Could you check a few things on this model? Use its own coordinates, in mm. A direction names the side the tool comes from. Round coordinates to 2 decimals unless told otherwise and drop trailing zeros. Write each loop counter-clockwise with the first axis right and the second up, starting at its lowest first coordinate (ties: lowest second). Pieces come first, ordered by that corner, then holes. Notation, with made-up numbers: (35.5, 7) -> (51.5, 7) arc R22 cw to (51.5, 46) -> close; hole circle Ø10 at (33.5, 69.5). An arc over 180 degrees is marked (long way). Answer in a Markdown table with one row per item. Add a question column.
```python
from build123d import *

# Parameters (mm, degrees)
F0_R     = 2
F1_DEPTH = 40
F3_DEPTH = 5
F5_DEPTH = 10
F6_W     = 0.9371294279
F6_H     = 2
F6_W_2   = 0.6703293088
F6_W_3   = 1
F7_DEPTH = 25


with BuildPart() as f1:
    # F0 (on Top) → F1 (new body)
    with BuildSketch(Plane.XY):
        Circle(F0_R)
    extrude(amount=F1_DEPTH)

    # F2 (on face) → F3 (join)
    with BuildSketch(Plane.XY.offset(40)):
        with BuildLine():
            Line((0, 2), (-1.1547005384, 2))
            Line((-1.1547005384, 2), (-1.7320507826, 1.0000000433))
            ThreePointArc((-1.7320507826, 1.0000000433), (-0.9999999783, 1.7320508201), (0, 2))
        make_face()
        with BuildLine():
            ThreePointArc((-1.7320507826, -1.0000000433), (-2, 0), (-1.7320507826, 1.0000000433))
            Line((-1.7320507826, 1.0000000433), (-2.3094010768, 0))
            Line((-2.3094010768, 0), (-1.7320507826, -1.0000000433))
        make_face()
        with BuildLine():
            ThreePointArc((0, -2), (-0.9999999783, -1.7320508201), (-1.7320507826, -1.0000000433))
            Line((-1.7320507826, -1.0000000433), (-1.1547005384, -2))
            Line((-1.1547005384, -2), (0, -2))
        make_face()
        with BuildLine():
            ThreePointArc((1.7320507983, -1.0000000161), (0.999999992, -1.7320508122), (0, -2))
            Line((0, -2), (1.1547005384, -2))
            Line((1.1547005384, -2), (1.7320507983, -1.0000000161))
        make_face()
        with BuildLine():
            Line((2.3094010768, 0), (1.7320507826, 1.0000000433))
            ThreePointArc((1.7320507826, 1.0000000433), (1.9318516461, 0.5176381144), (2, 0))
            ThreePointArc((2, 0), (1.9318516502, -0.5176380992), (1.7320507983, -1.0000000161))
            Line((1.7320507983, -1.0000000161), (2.3094010768, 0))
        make_face()
        with BuildLine():
            Line((1.1547005384, 2), (0, 2))
            ThreePointArc((0, 2), (0.9999999783, 1.7320508201), (1.7320507826, 1.0000000433))
            Line((1.7320507826, 1.0000000433), (1.1547005384, 2))
        make_face()
        with BuildLine():
            ThreePointArc((1.7320507826, 1.0000000433), (0.9999999783, 1.7320508201), (0, 2))
            ThreePointArc((0, 2), (-0.9999999783, 1.7320508201), (-1.7320507826, 1.0000000433))
            ThreePointArc((-1.7320507826, 1.0000000433), (-2, 0), (-1.7320507826, -1.0000000433))
            ThreePointArc((-1.7320507826, -1.0000000433), (-0.9999999783, -1.7320508201), (0, -2))
            ThreePointArc((0, -2), (0.999999992, -1.7320508122), (1.7320507983, -1.0000000161))
            ThreePointArc((1.7320507983, -1.0000000161), (1.9318516502, -0.5176380992), (2, 0))
            ThreePointArc((2, 0), (1.9318516461, 0.5176381144), (1.7320507826, 1.0000000433))
        make_face()
    extrude(amount=F3_DEPTH)

    # F4 (on face) → F5 (join)
    with BuildSketch(Plane(origin=(0, 0, 0), x_dir=(1, 0, 0), z_dir=(0, 0, -1))):
        with BuildLine():
            ThreePointArc((1.1, 1.6703293088), (0.5741695665, 1.915810353), (0, 2))
            ThreePointArc((0, 2), (-0.5741695665, 1.915810353), (-1.1, 1.6703293088))
            Line((-1.1, 1.6703293088), (-1.1, -1.6703293088))
            ThreePointArc((-1.1, -1.6703293088), (-0.5741695665, -1.915810353), (0, -2))
            ThreePointArc((0, -2), (0.5741695665, -1.915810353), (1.1, -1.6703293088))
            Line((1.1, -1.6703293088), (1.1, 1.6703293088))
        make_face()
    extrude(amount=F5_DEPTH)

    # F6 (on face) → F7 (cut)
    with BuildSketch(Plane.YZ.offset(1.1)):
        with Locations((-2.1388940228, -4.197623184)):
            Rectangle(F6_W, F6_H)
        with Locations((-1.3351646544, -4.197623184)):
            Rectangle(F6_W_2, F6_H)
        with Locations((-0.5, -4.197623184)):
            Rectangle(F6_W_3, F6_H)
        with BuildLine():
            Line((1, -3.197623184), (0, -3.197623184))
            Line((0, -3.197623184), (0, -5.197623184))
            Line((0, -5.197623184), (-1, -5.197623184))
            Line((-1, -5.197623184), (-1, -6.7451779507))
            ThreePointArc((-1, -6.7451779507), (-0.7071067812, -7.4522847319), (0, -7.7451779507))
            ThreePointArc((0, -7.7451779507), (0.7071067812, -7.4522847319), (1, -6.7451779507))
            Line((1, -6.7451779507), (1, -3.197623184))
        make_face()
    extrude(amount=-F7_DEPTH, mode=Mode.SUBTRACT)


solid = f1.part
```
(1) On a 3-axis mill with a long thin cutter (end or side, diameter ignored), from which of +Z, -Z, +X, -X, +Y, -Y can I reach the whole of each face in a straight line? I mean faces 1 (the face through (-1.1, 1.5, -4.9)), 2 (the face through (0, 0, -3.198)), 3 (the face through (1.4, 0, 0)), 4 (the face through (0, -1, -6)). Say none if no direction works.
(2) Suppose I cut it at A-A, the plane z = 10. Please give me the cut outline in (x, y).
(3) If we mould it in two halves opening along Y, with no side actions, what happens to faces 5 (the face through (0, 1, -5)), 6 (the face through (-1.5, 0, 0)), 7 (the face through (0, 2, 42)), 8 (the face through (0, -2, 42))? For each: pulls with the +Y half, pulls with the -Y half, needs draft (parallel to the pull), parting line crosses it, or undercut.
(4) For P1, Ø1.2, axis at x = 0.5, z = -6, coming from the +Y side; P2, Ø0.5, axis at x = -2, y = 0, coming from the -Z side; P3, Ø1.5, axis at y = -1, z = 32.5, coming from the -X side; P4, Ø0.7, axis at x = 0.5, z = -4.5, coming from the -Y side, each with a flat end and sliding along its axis, tell me the tip position at first contact or that it passes through.
(5) I need wall thicknesses on L1, parallel to Z at x = -0.8, y = -0.1; L2, parallel to Y at x = -1, z = -5.5; L3, parallel to Z at x = 0.75, y = -1.7. Which ranges of each line are inside material? Lowest first, please.
Response:
| question | item | result |
|---|---|---|
| 1 | face 1 | -Z, -X, +Y, -Y |
| 1 | face 2 | +X, -X, -Y |
| 1 | face 3 | -Z, +X, +Y, -Y |
| 1 | face 4 | +X, -X |
| 2 | outline | circle Ø4 at (0, 0) |
| 3 | face 5 | undercut |
| 3 | face 6 | needs draft |
| 3 | face 7 | pulls with the +Y half |
| 3 | face 8 | pulls with the -Y half |
| 4 | P1 | y = 2 |
| 4 | P2 | z = 0 |
| 4 | P3 | x = -1.98 |
| 4 | P4 | y = 1 |
| 5 | L1 | -10 to -7.74, -3.2 to 45 |
| 5 | L2 | -1.73 to -1, 1 to 1.73 |
| 5 | L3 | -10 to -5.2, -3.2 to 45 |
